The model under review builds one solid part; all positions refer to its coordinate system, in mm. Face numbers are marked on the shaded views. A direction names the side the tool comes from. Round coordinates to 2 decimals unless told otherwise and drop trailing zeros. Order: outer loops, then holes, each group sorted by start corner. A loop starts at its lowest first (then second) coordinate and runs counter-clockwise, first axis right, second up. Notation, with made-up numbers: (22, 1.5) - (77, 1.5) arc R21 cw to (77, 18.5) - close; hole circle Ø3 at (51.5, -10). An arc over 180 degrees is marked (long way). One line per question, with ' | ' between items. Start each with the question number.
Item 1: Add section D-D on y = 60. State the section outline as (x, z) points, and give its area (3 significant figures).
Item 2: Draft analysis for pull direction X (two halves, no side actions). For the marked faces 1, 2, 3 and 4, state which applies: +X half, -X half, draft (parallel to the pull), parting line (faces both ways), or undercut.
Item 3: Insertion check: pin 1 Ø2 at (y, z) = (23.5, -84.5) entering from +X; pin 2 Ø5 at (x, y) = (-66.5, 20) entering from -Z; pin 3 Ø10 at (y, z) = (53.5, -82) entering from -X; pin 4 Ø6 at (x, z) = (-12.7, -12.7) entering from +Y. Each pin has a flat end and moves straight along its axis. Give the tip position at first contact, or say it passes through.
Item 4: For L1, parallel to Y at x = -61.5, z = -29; L2, parallel to Z at x = -62, y = 10; L3, parallel to Z at x = -45.5, y = 42, list the stretches that pass through material, from the lowest coordinate up. Write a range as [from, to].
Item 5: Add section B-B on z = -21. State the section outline as (x, y) points.
Item 6: Add section C-C on x = -4.5. State the section outline as (y, z) points.
Item 7: Tool access review of the marked faces 5 and 6: name each direction out of +Z, -Z, +X, -X, +Y, -Y from which nothing blocks a thin tool from reaching the whole face with its end or side.
Item 8: Add section A-A on x = -65.5. State the section outline as (y, z) points, and give its area (3 significant figures).
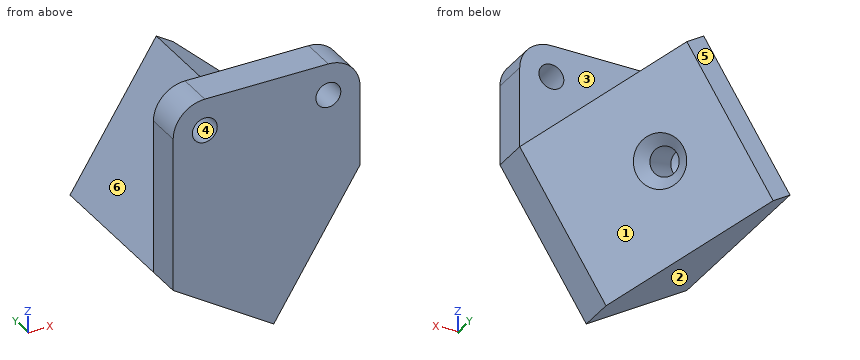
from build123d import *

# Parameters (mm, degrees)
BASE_EXTRUDE_DEPTH                               = 14.2875
BOSS_EXTRUDE1_DEPTH                              = 60.325
CUT_EXTRUDE1_DEPTH                               = 115.691718555
CSK_FOR_M10_FLAT_HEAD_MACHINE_SCREW1_D           = 11
CSK_FOR_M10_FLAT_HEAD_MACHINE_SCREW1_DEPTH       = 25.4
CSK_FOR_M10_FLAT_HEAD_MACHINE_SCREW1_CSINK_D     = 20
CSK_FOR_M10_FLAT_HEAD_MACHINE_SCREW1_CSINK_ANGLE = 90
CSK_FOR_M10_FLAT_HEAD_MACHINE_SCREW1_TIP         = 3.304733405
FILLET1_R                                        = 12.7
F_10_0_10_DIAMETER_HOLE1_D                       = 10


with BuildPart() as part:
    # Sketch1 → Base-Extrude (new body)
    with BuildSketch(Plane(origin=(0, 0, 0), x_dir=(1, 0, 0), z_dir=(0, 1, 0))):
        Polygon((0, 0), (0, 45), (-34.641016151, 100), (-75, 74.580432521), (-75, 0), align=None)
    extrude(amount=BASE_EXTRUDE_DEPTH)

    # Sketch2 → Boss-Extrude1 (add)
    with BuildSketch(Plane(origin=(0, 14.2875, 0), x_dir=(-1, 0, 0), z_dir=(0, 1, 0))):
        Polygon((34.641016151, -100), (75, -74.580432521), (40.358983849, -19.580432521), (0, -45), align=None)
    extrude(amount=BOSS_EXTRUDE1_DEPTH)

    # Sketch3 → Cut-Extrude1 (cut, through all)
    with BuildSketch(Plane(origin=(-20.292666266, 0, -32.218934911), x_dir=(0.846153846153846, 0, -0.5329387100211933), z_dir=(0.5329387100211932, 0, 0.8461538461538459))):
        Polygon((-138.006469686, 260.451535778), (-15.714738961, 74.6125), (23.982241951, 14.2875), (146.273972676, -171.551535778), (517.952044233, 73.031925672), (233.67160187, 505.034997229), align=None)
    extrude(amount=-CUT_EXTRUDE1_DEPTH, mode=Mode.SUBTRACT)

    # CSK for M10 Flat Head Machine Screw1
    with Locations(Plane(origin=(19.712140487, 15.330086336, -12.415428673), x_dir=(-0.36778462315379085, -0.25201220679427455, -0.8951113442462362), z_dir=(0.7068403651551289, 0.549708126864638, -0.4451939728324442))):
        with Locations((53.6091088, 60.43353944)):
            CounterSinkHole(CSK_FOR_M10_FLAT_HEAD_MACHINE_SCREW1_D / 2, CSK_FOR_M10_FLAT_HEAD_MACHINE_SCREW1_CSINK_D / 2, depth=CSK_FOR_M10_FLAT_HEAD_MACHINE_SCREW1_DEPTH, counter_sink_angle=CSK_FOR_M10_FLAT_HEAD_MACHINE_SCREW1_CSINK_ANGLE)
            with Locations((0, 0, -(CSK_FOR_M10_FLAT_HEAD_MACHINE_SCREW1_DEPTH + CSK_FOR_M10_FLAT_HEAD_MACHINE_SCREW1_TIP / 2))):  # 118° drill point
                Cone(0, CSK_FOR_M10_FLAT_HEAD_MACHINE_SCREW1_D / 2, CSK_FOR_M10_FLAT_HEAD_MACHINE_SCREW1_TIP, mode=Mode.SUBTRACT)

    # Fillet1
    fillet1_edges = [part.edges().sort_by_distance(p)[0] for p in [
        (0, 7.14375, 0),
        (-75, 7.14375, 0),
    ]]
    fillet(fillet1_edges, radius=FILLET1_R)

    # Ø10.0 (10) Diameter Hole1 (through all)
    with Locations(Plane(origin=(0, 14.2875, 0), x_dir=(-1, 0, 0), z_dir=(0, 1, 0))):
        with Locations((12.7, -12.7), (62.3, -12.7)):
            Hole(F_10_0_10_DIAMETER_HOLE1_D / 2)


solid = part.part
Determined:
1) outline: (-75, -74.58) - (-60.09, -83.97) - (-25.45, -28.97) - (-40.36, -19.58) - close | area: 1,150 mm2
2) face 1: +X half | face 2: -X half | face 3: draft | face 4: undercut
3) pin 1: x = -31.04 | pin 2: z = -81.51 | pin 3: x = -71.16 | pin 4: through
4) L1: [0, 14.29] | L2: [-82.77, -17.69], [-7.71, 0] | L3: [-83.02, -59.08], [-46.92, -27.74]
5) outline: (-75, 0) - (0, 0) - (0, 14.29) - (-38.11, 14.29) - (-38.11, 74.61) - (-41.25, 74.61) - (-41.25, 14.29) - (-75, 14.29) - close
6) outline: (0, -52.14) - (14.29, -52.14) - (22.37, -42.17) - (14.29, -42.17) - (14.29, -3) - (0, -3) - close
7) face 5: +Z, -Z, +X, -X, +Y | face 6: +Z, -X, +Y
8) outline: (0, -80.56) - (69.71, -80.56) - (74.61, -74.51) - (74.61, -59.5) - (14.29, -59.5) - (14.29, -16.54) - (0, -16.54) - close; (0, -8.86) - (14.29, -8.86) - (14.29, -0.41) - (0, -0.41) - close | area: 2,290 mm2
